Input: part model. Units: mm. Frame: model coordinates. A direction names the side the tool comes from. Coordinates: 2 decimals unless noted, no trailing zeros. Write each loop counter-clockwise with the first axis right and the second up, starting at its lowest first coordinate (ties: lowest second). Pieces come first, ordered by that corner, then holes. Notation, with made-up numbers: M -36,19.5 L -22,19.5 A23 cw -22,42.5 Z; hole C 11,-8.75 d6. An arc over 180 degrees is marked long. Use one line per item in the form item = value.
from build123d import *

# Parameters (mm, degrees)
SKETCH1_R                    = 11.1125
BOSS_EXTRUDE1_DEPTH          = 7.14375
CHAMFER1_SIZE                = 0.508
F_3_8_0_375_DIAMETER_HOLE1_D = 9.525
SKETCH5_R                    = 9.2075
SKETCH5_R_2                  = 6.6675
CUT_EXTRUDE1_DEPTH           = 0.254
CUT_EXTRUDE2_START           = -0.254
SKETCH6_R                    = 9.2075
SKETCH6_R_2                  = 6.6675
CUT_EXTRUDE2_DEPTH           = 0.254


with BuildPart() as part:
    # Sketch1 → Boss-Extrude1 (new body)
    with BuildSketch(Plane.XY):
        Circle(SKETCH1_R)
    extrude(amount=BOSS_EXTRUDE1_DEPTH)

    # Chamfer1
    chamfer1_edges = [part.edges().sort_by_distance(p)[0] for p in [
        (-11.1125, 0, 0),
        (-11.1125, 0, 7.14375),
    ]]
    chamfer(chamfer1_edges, length=CHAMFER1_SIZE)

    # 3/8 (0.375) Diameter Hole1 (through all)
    with Locations(Plane.XY.offset(7.14375)):
        with Locations((0, 0)):
            Hole(F_3_8_0_375_DIAMETER_HOLE1_D / 2)

    # Sketch5 → Cut-Extrude1 (cut)
    with BuildSketch(Plane.XY.offset(7.14375)):
        Circle(SKETCH5_R)
        Circle(SKETCH5_R_2, mode=Mode.SUBTRACT)
    extrude(amount=-CUT_EXTRUDE1_DEPTH, mode=Mode.SUBTRACT)

    # Sketch6 → Cut-Extrude2 (cut)
    with BuildSketch(Plane(origin=(0, 0, 0), x_dir=(-1, 0, 0), z_dir=(0, 0, -1)).offset(CUT_EXTRUDE2_START)):
        with Locations(Location((0, 0, 0), (0, 0, 180))):
            Circle(SKETCH6_R)
        with Locations(Location((0, 0, 0), (0, 0, 180))):
            Circle(SKETCH6_R_2, mode=Mode.SUBTRACT)
    extrude(amount=CUT_EXTRUDE2_DEPTH, mode=Mode.SUBTRACT)


solid = part.part
(1) Section query C-C on z = 4.75. Return the cut outline in (x, y) (1 decimal), plus the area to 3 significant figures.
Computed:
outline = C 0,0 d22.2; hole C 0,0 d9.5
area = 317 mm^2
(2) Set-up query: faces 1 (the flat face through (5, -5, 0.254)), 2 (the flat face through (-3, 9, 0)), 3 (the flat face through (5, 5, 6.89)). Return all of +Z, -Z, +X, -X, +Y, -Y with unobstructed straight access to the full face (end or side cutting, diameter ignored); none if empty.
Computed:
face_1 = -Z
face_2 = -Z, +X, -X, +Y, -Y
face_3 = +Z
(3) Section query A-A on y = 0. Return the cut outline in (x, z).
Computed:
outline = M -11.11,0.51 L -10.6,0 L -9.21,0 L -9.21,0.25 L -6.67,0.25 L -6.67,0 L -4.76,0 L -4.76,7.14 L -6.67,7.14 L -6.67,6.89 L -9.21,6.89 L -9.21,7.14 L -10.6,7.14 L -11.11,6.64 Z; M 4.76,0 L 6.67,0 L 6.67,0.25 L 9.21,0.25 L 9.21,0 L 10.6,0 L 11.11,0.51 L 11.11,6.64 L 10.6,7.14 L 9.21,7.14 L 9.21,6.89 L 6.67,6.89 L 6.67,7.14 L 4.76,7.14 Z
(4) First-contact query: pin 1 Ø8.5 at (x, y) = (0, 0) entering from +Z. Flat tip, straight axial feed; report the tip coordinate or a pass-through.
Computed:
pin_1 = through
(5) Line query: probe 1 along Y at (x, z) = (0, 5.5); probe 2 along Z at (x, y) = (3.25, 6.75); probe 3 along Y at (x, z) = (1, 5.5). Output: solid intervals per line, ascending.
Computed:
probe_1 = -11.11 to -4.76, 4.76 to 11.11
probe_2 = 0.25 to 6.89
probe_3 = -11.07 to -4.66, 4.66 to 11.07
